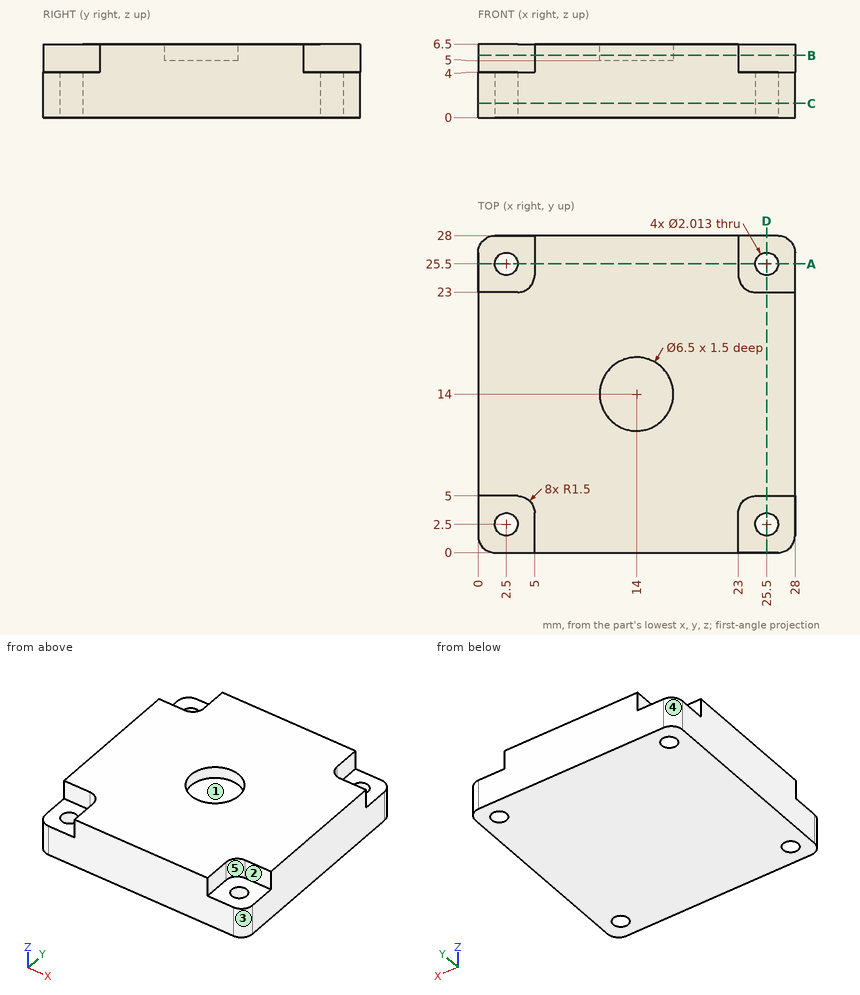
The figure shows three views and two pictorial views of one solid part (mm, origin at its lowest corner). Answer the questions. A direction names the side the tool comes from. Coordinates: 2 decimals unless noted, no trailing zeros. Loops run counter-clockwise (first coordinate to the right, second up) from the corner with the lowest first, then second, coordinate; pieces in that order, holes last. Notation, with made-up numbers: (20.5, 22.25) -> (43.5, 22.25) arc R21 ccw to (43.5, 60.25) -> close; hole circle Ø11 at (35.5, -19). An arc over 180 degrees is marked (long way). Return JSON: item names as keys, results as strings. Group by question number.
(1) A cutting plane is placed at C-C on z = 1.25. Write down the section's boundary in (x, y).
(2) A cutting plane is placed at B-B on z = 5.5. Write down the section's boundary in (x, y), and give its area (3 significant figures).
(3) Given pin 1 Ø3 at (x, y) = (25.5, 25.5) entering from +Z; pin 2 Ø3 at (x, y) = (13, 13.5) entering from +Z; pin 3 Ø2 at (x, z) = (2.5, 6) entering from +Y; pin 4 Ø1.8 at (x, y) = (2.5, 25.5) entering from -Z, each flat-ended and moving along its own axis, determine where each tip first touches the part or whether it passes through.
(4) Determine the mould class of the marked faces 1, 2 and 3 for opening direction X: released by +X, released by -X, zero draft, split by the parting line, or undercut.
(5) A cutting plane is placed at A-A on y = 25.5. Write down the section's boundary in (x, z), and give its area (3 significant figures).
(6) Find the intervals of material crossed by probe 1 along X at (y, z) = (2.5, 2.9); probe 2 along Z at (x, y) = (26.5, 4.5), in increasing order. Write a range as from..to.
(7) Which of the six approach directions +Z, -Z, +X, -X, +Y, -Y give full straight-line access (tool end or side, diameter ignored) to the marked faces 4 and 5?
The answers:
{
 "1": {"outline": "(0, 1.5) arc R1.5 ccw to (1.5, 0) -> (26.5, 0) arc R1.5 ccw to (28, 1.5) -> (28, 26.5) arc R1.5 ccw to (26.5, 28) -> (1.5, 28) arc R1.5 ccw to (0, 26.5) -> close; hole circle Ø2.01 at (2.5, 2.5); hole circle Ø2.01 at (2.5, 25.5); hole circle Ø2.01 at (25.5, 2.5); hole circle Ø2.01 at (25.5, 25.5)"},
 "2": {"outline": "(0, 5) -> (3.5, 5) arc R1.5 cw to (5, 3.5) -> (5, 0) -> (23, 0) -> (23, 3.5) arc R1.5 cw to (24.5, 5) -> (28, 5) -> (28, 23) -> (24.5, 23) arc R1.5 cw to (23, 24.5) -> (23, 28) -> (5, 28) -> (5, 24.5) arc R1.5 cw to (3.5, 23) -> (0, 23) -> close; hole circle Ø6.5 at (14, 14)", "area": "653 mm^2"},
 "3": {"pin 1": "stops at z = 4", "pin 2": "stops at z = 5", "pin 3": "stops at y = 23", "pin 4": "passes through"},
 "4": {"face 1": "undercut", "face 2": "zero draft", "face 3": "released by +X"},
 "5": {"outline": "(0, 0) -> (1.49, 0) -> (1.49, 4) -> (0, 4) -> close; (3.51, 0) -> (24.49, 0) -> (24.49, 4) -> (23, 4) -> (23, 6.5) -> (5, 6.5) -> (5, 4) -> (3.51, 4) -> close; (26.51, 0) -> (28, 0) -> (28, 4) -> (26.51, 4) -> close", "area": "141 mm^2"},
 "6": {"probe 1": "x = 0..1.49, 3.51..24.49, 26.51..28", "probe 2": "z = 0..4"},
 "7": {"face 4": "+Z, -Z, -X, +Y", "face 5": "+Z, +X, -Y"}
}
